Geometry: final body of the model. Coordinates: model frame, mm. A direction names the side the tool comes from. Round coordinates to 2 decimals unless told otherwise and drop trailing zeros. Write each loop counter-clockwise with the first axis right and the second up, starting at its lowest first coordinate (ties: lowest second). Pieces come first, ordered by that corner, then holes.
from build123d import *

# Parameters (mm, degrees)
CUT_EXTRUDE1_DEPTH      = 59.259372654
CUT_EXTRUDE1_DEPTH_BACK = 59.259372654
SKETCH2_R               = 1.9812
CHAMFER1_SIZE           = 0.8128
CHAMFER2_SIZE           = 0.635


with BuildPart() as part:
    # Sketch4 → Revolve1 (revolve)
    with BuildSketch(Plane(origin=(0, 0, 0), x_dir=(0, 0, -1), z_dir=(1, 0, 0)), mode=Mode.PRIVATE) as revolve1_sk:
        Polygon((-4.064, 0), (50.8, 0), (50.8, 6.35), (0, 6.35), (0, 8.001), (-4.064, 8.001), align=None)
    revolve(revolve1_sk.sketch.rotate(Axis((0, 0, 4.064), (0, 0, -1)), 180), axis=Axis((0, 0, 4.064), (0, 0, -1)))

    # Sketch2 → Cut-Extrude1 (cut, two sides: drawn at the far end of the back side and taken through both)
    with BuildSketch(Plane(origin=(0, 0, 6.35), x_dir=(0, 0, 1), z_dir=(-1, 0, 0)).offset(-CUT_EXTRUDE1_DEPTH_BACK)):
        with Locations((-52.7812, 0)):
            Circle(SKETCH2_R)
    extrude(amount=CUT_EXTRUDE1_DEPTH + CUT_EXTRUDE1_DEPTH_BACK, mode=Mode.SUBTRACT)

    # Chamfer1
    chamfer1_edges = [part.edges().sort_by_distance(p)[0] for p in [
        (0, 8.001, 4.064),
    ]]
    chamfer(chamfer1_edges, length=CHAMFER1_SIZE)

    # Chamfer2
    chamfer2_edges = [part.edges().sort_by_distance(p)[0] for p in [
        (0, 6.35, -50.8),
    ]]
    chamfer(chamfer2_edges, length=CHAMFER2_SIZE)


solid = part.part
1) Section B-B on y = 0. Output: boundary loops of the cut face in (x, z) (3 decimals).
2) Reachability of faces 1 (the cylindrical face through (7.81, 1.73, 1.65)), 2 (the cylindrical face through (-1.907, -6.057, -24.731)) from +Z, -Z, +X, -X, +Y, -Y: full face, straight path, thin tool, end or side. Return the list, or none.
3) Draft query along Z for faces 3 (the flat face through (0, 0, 4.064)), 4 (the flat face through (0, 0, -50.8)), 5 (the cylindrical face through (0.09, -0.76, -44.6)). Return one class per face: pulls with the +Z half, pulls with the -Z half, needs draft (parallel to the pull), parting line crosses it, or undercut.
4) Section C-C on z = -24. Output: boundary loops of the cut face in (x, y).
5) Section A-A on x = 0. Output: boundary loops of the cut face in (y, z) (3 decimals).
6) Line query: probe 1 along Z at (x, y) = (3.25, 0); probe 2 along Z at (x, y) = (0.25, -0.75); probe 3 along Z at (x, y) = (-3.75, -5.25). Output: solid intervals per line, ascending.
7) First-contact query: P1, Ø4, axis at x = 5.5, z = -18.5, coming from the +Y side; P2, Ø8, axis at y = -1, z = -36, coming from the +X side; P3, Ø8, axis at x = 4, z = -21.5, coming from the -Y side. Flat tips, straight axial feed; report the tip coordinate or a pass-through.
Filled in:
1. outline: (-8.001, 0) - (-6.35, 0) - (-6.35, -44.45) - (6.35, -44.45) - (6.35, 0) - (8.001, 0) - (8.001, 3.251) - (7.188, 4.064) - (-7.188, 4.064) - (-8.001, 3.251) - close; (-6.35, -50.165) - (-5.715, -50.8) - (5.715, -50.8) - (6.35, -50.165) - (6.35, -48.412) - (-6.35, -48.412) - close
2. face 1: +Z, -Z
2. face 2: -Z
3. face 3: pulls with the +Z half
3. face 4: pulls with the -Z half
3. face 5: undercut
4. outline: circle Ø12.7 at (0, 0)
5. outline: (-8.001, 0) - (-6.35, 0) - (-6.35, -50.165) - (-5.715, -50.8) - (5.715, -50.8) - (6.35, -50.165) - (6.35, 0) - (8.001, 0) - (8.001, 3.251) - (7.188, 4.064) - (-7.188, 4.064) - (-8.001, 3.251) - close; hole circle Ø3.962 at (0, -46.431)
6. probe 1: z = -50.8 to -48.41, -44.45 to 4.06
6. probe 2: z = -50.8 to -48.26, -44.6 to 4.06
6. probe 3: z = 0 to 4.06
7. P1: stops at y = 5.3
7. P2: stops at x = 6.35
7. P3: stops at y = -6.35
